```python
from build123d import *

# Parameters (mm, degrees)
ESQUISSE2_W                                        = 150
ESQUISSE2_H                                        = 80
BOSS_EXTRU_1_DEPTH                                 = 6
CHAMBRAGE_POUR_VIS_T_TE_HEXAGONALE_M31_D           = 3.4
CHAMBRAGE_POUR_VIS_T_TE_HEXAGONALE_M31_DEPTH       = 15
CHAMBRAGE_POUR_VIS_T_TE_HEXAGONALE_M31_CBORE_D     = 6.5
CHAMBRAGE_POUR_VIS_T_TE_HEXAGONALE_M31_CBORE_DEPTH = 3.4
CHAMBRAGE_POUR_VIS_T_TE_HEXAGONALE_M31_TIP         = 1.021463052
ENL_V_MAT_EXTRU_2_DEPTH                            = 4
ENL_V_MAT_EXTRU_3_DEPTH                            = 171.1058494
ENL_V_MAT_EXTRU_4_DEPTH                            = 4
ENL_V_START                                        = -4
ENL_V_MAT_EXTRU_5_DEPTH                            = 4


with BuildPart() as part:
    # Esquisse2 → Boss.-Extru.1 (new body)
    with BuildSketch(Plane(origin=(0, 0, 0), x_dir=(1, 0, 0), z_dir=(0, 1, 0))):
        with Locations((75, 40)):
            Rectangle(ESQUISSE2_W, ESQUISSE2_H)
    extrude(amount=BOSS_EXTRU_1_DEPTH)

    # Chambrage pour vis à tête hexagonale M31
    with Locations(Plane(origin=(90, 0, -67), x_dir=(0, 0, -1), z_dir=(0, -1, 0))):
        with Locations((0, 0), (0, -30), (-57, -39.25), (-57, 9.25)):
            CounterBoreHole(CHAMBRAGE_POUR_VIS_T_TE_HEXAGONALE_M31_D / 2, CHAMBRAGE_POUR_VIS_T_TE_HEXAGONALE_M31_CBORE_D / 2, CHAMBRAGE_POUR_VIS_T_TE_HEXAGONALE_M31_CBORE_DEPTH, depth=CHAMBRAGE_POUR_VIS_T_TE_HEXAGONALE_M31_DEPTH)
            with Locations((0, 0, -(CHAMBRAGE_POUR_VIS_T_TE_HEXAGONALE_M31_DEPTH + CHAMBRAGE_POUR_VIS_T_TE_HEXAGONALE_M31_TIP / 2))):  # 118° drill point
                Cone(0, CHAMBRAGE_POUR_VIS_T_TE_HEXAGONALE_M31_D / 2, CHAMBRAGE_POUR_VIS_T_TE_HEXAGONALE_M31_TIP, mode=Mode.SUBTRACT)

    # Esquisse6 → Enlèv. mat.-Extru.2 (cut)
    with BuildSketch(Plane.XZ):
        with BuildLine():
            Line((90, -71.278666631), (60, -71.278666631))
            ThreePointArc((60, -71.278666631), (55.721333369, -67), (60, -62.721333369))
            Line((60, -62.721333369), (90, -62.721333369))
            ThreePointArc((90, -62.721333369), (94.278666631, -67), (90, -71.278666631))
        make_face()
    extrude(amount=-ENL_V_MAT_EXTRU_2_DEPTH, mode=Mode.SUBTRACT)

    # Esquisse7 → Enlèv. mat.-Extru.3 (cut, through all)
    with BuildSketch(Plane.XZ):
        with BuildLine():
            Line((90, -68.7), (60, -68.7))
            ThreePointArc((60, -68.7), (58.3, -67), (60, -65.3))
            Line((60, -65.3), (90, -65.3))
            ThreePointArc((90, -65.3), (91.7, -67), (90, -68.7))
        make_face()
    extrude(amount=-ENL_V_MAT_EXTRU_3_DEPTH, mode=Mode.SUBTRACT)

    # Esquisse9 → Enlèv. mat.-Extru.4 (cut)
    with BuildSketch(Plane(origin=(0, 0, 0), x_dir=(-1, 0, 0), z_dir=(0, -1, 0))):
        with BuildLine():
            Line((-102.5, 13.5), (-47.5, 13.5))
            ThreePointArc((-47.5, 13.5), (-44, 10), (-47.5, 6.5))
            Line((-47.5, 6.5), (-102.5, 6.5))
            ThreePointArc((-102.5, 6.5), (-106, 10), (-102.5, 13.5))
        make_face()
    extrude(amount=-ENL_V_MAT_EXTRU_4_DEPTH, mode=Mode.SUBTRACT)

    # Esquisse10 → Enlèv. mat.-Extru.5 (cut)
    with BuildSketch(Plane(origin=(0, 4, 0), x_dir=(-1, 0, 0), z_dir=(0, -1, 0)).offset(ENL_V_START)):
        with BuildLine():
            Line((-99.25, 11.7), (-50.75, 11.7))
            ThreePointArc((-50.75, 11.7), (-49.05, 10), (-50.75, 8.3))
            Line((-50.75, 8.3), (-99.25, 8.3))
            ThreePointArc((-99.25, 8.3), (-100.95, 10), (-99.25, 11.7))
        make_face()
    extrude(amount=ENL_V_MAT_EXTRU_5_DEPTH, mode=Mode.SUBTRACT)


solid = part.part
```
Work out the finished part from the listing and answer in its coordinate system (mm). A direction names the side the tool comes from. Round coordinates to 2 decimals unless told otherwise and drop trailing zeros. Write each loop counter-clockwise with the first axis right and the second up, starting at its lowest first coordinate (ties: lowest second). Pieces come first, ordered by that corner, then holes.
1) Determine the mould class of faces 3 (the face through (74, 0, -41)), 4 (the face through (75, 2, -6.5)), 5 (the face through (0, 3, -39)) for opening direction X: pulls with the +X half, pulls with the -X half, needs draft (parallel to the pull), parting line crosses it, or undercut.
2) A cutting plane is placed at B-B on x = 86. Determine the outline of the cut face in (y, z), and give its area (3 significant figures).
3) Consider probe 1 along Z at (x, y) = (66, 0.95); probe 2 along Z at (x, y) = (75.5, 4.1); probe 3 along Z at (x, y) = (53.5, 0.9). Determine where each line is inside the solid, lowest interval first.
4) A cutting plane is placed at D-D on z = -67. Determine the outline of the cut face in (x, y).
5) Flat-ended cylindrical pins translate along their axes: P1, Ø5, axis at x = 117, z = -19, coming from the -Y side; P2, Ø2, axis at x = 73, z = -10.5, coming from the -Y side. Find the tip coordinate at first contact, or state that the pin passes through.
6) Which of the six approach directions +Z, -Z, +X, -X, +Y, -Y give full straight-line access (tool end or side, diameter ignored) to faces 1 (the face through (150, 3, -39)), 2 (the face through (75, 4, -69))?
7) A cutting plane is placed at A-A on z = -10. Determine the outline of the cut face in (x, y).
8) A cutting plane is placed at C-C on y = 2.7. Determine the outline of the cut face in (x, z), and give its area (3 significant figures).
Entries:
1. face 3: needs draft
1. face 4: undercut
1. face 5: pulls with the -X half
2. outline: (0, -80) - (6, -80) - (6, -68.7) - (4, -68.7) - (4, -71.28) - (0, -71.28) - close; (0, -62.72) - (4, -62.72) - (4, -65.3) - (6, -65.3) - (6, -11.7) - (4, -11.7) - (4, -13.5) - (0, -13.5) - close; (0, -6.5) - (4, -6.5) - (4, -8.3) - (6, -8.3) - (6, 0) - (0, 0) - close
2. area: 404 mm2
3. probe 1: z = -80 to -71.28, -62.72 to -13.5, -6.5 to 0
3. probe 2: z = -80 to -68.7, -65.3 to -11.7, -8.3 to 0
3. probe 3: z = -80 to -13.5, -6.5 to 0
4. outline: (0, 0) - (55.72, 0) - (55.72, 4) - (58.3, 4) - (58.3, 6) - (0, 6) - close; (91.7, 4) - (94.28, 4) - (94.28, 0) - (150, 0) - (150, 6) - (91.7, 6) - close
5. P1: stops at y = 0
5. P2: passes through
6. face 1: +Z, -Z, +X, +Y, -Y
6. face 2: -Y
7. outline: (0, 0) - (44, 0) - (44, 4) - (49.05, 4) - (49.05, 6) - (0, 6) - close; (100.95, 4) - (106, 4) - (106, 0) - (150, 0) - (150, 6) - (100.95, 6) - close
8. outline: (0, -80) - (150, -80) - (150, 0) - (0, 0) - close; hole (47.5, -13.5) - (102.5, -13.5) arc R3.5 ccw to (102.5, -6.5) - (47.5, -6.5) arc R3.5 ccw to start; hole (60, -71.28) - (90, -71.28) arc R4.28 ccw to (90, -62.72) - (60, -62.72) arc R4.28 ccw to start
8. area: 11,300 mm2
